For this review, use the dimensioned drawing (mm, ordinates from the lowest corner) and the shaded views. A direction names the side the tool comes from. Give positions to 0.01 mm unless a question says otherwise; leave off trailing zeros. Write each loop counter-clockwise with the first axis right and the second up, starting at its lowest first coordinate (ties: lowest second). Pieces come first, ordered by that corner, then holes.
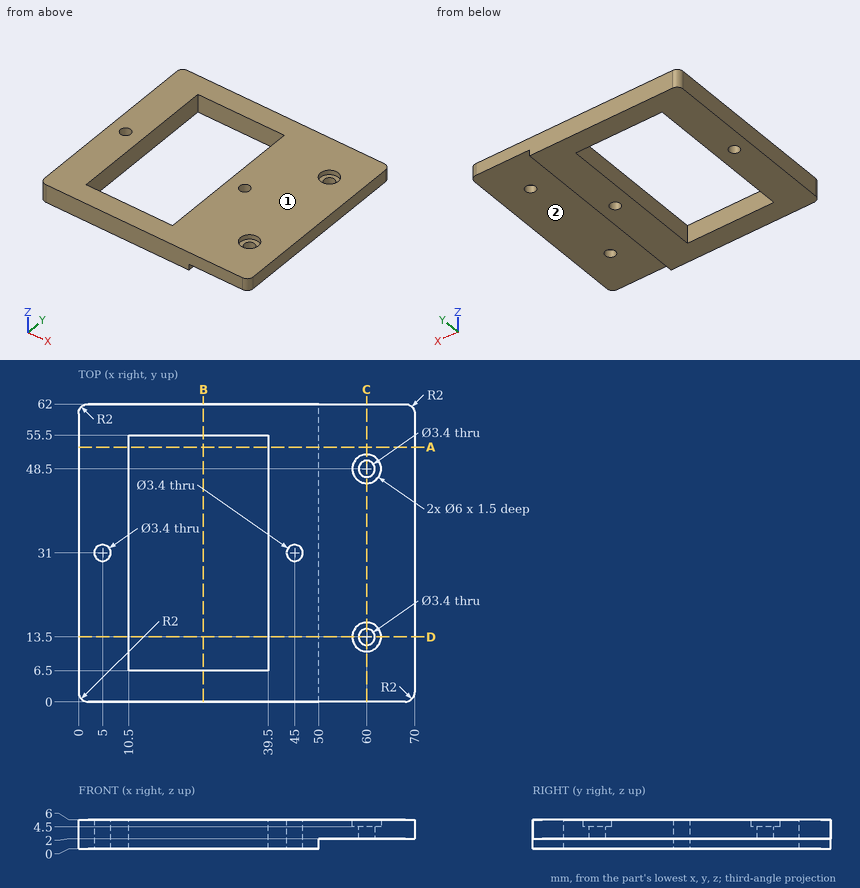
(1) We need section A-A (y = 53). Write out the cut boundary in (x, z), and give its area (3 significant figures).
(2) Tool access review of the marked faces 1 and 2: name each direction out of +Z, -Z, +X, -X, +Y, -Y from which nothing blocks a thin tool from reaching the whole face with its end or side.
(3) Clearance check with flat-ended pins moving along their axes: pin 1 Ø4.5 at (x, y) = (60, 13.5) entering from -Z; pin 2 Ø0.6 at (y, z) = (17.5, 0.5) entering from +X; pin 3 Ø1.8 at (x, y) = (61, 13) entering from +Z; pin 4 Ø3 at (x, y) = (5, 31) entering from -Z. State where each tip first meets the part, or that it passes through.
(4) For L1, parallel to Y at x = 60, z = 2.5; L2, parallel to Y at x = 60, z = 4.95; L3, parallel to Y at x = 27.5, z = 5.35, list the stretches that pass through material, from the lowest coordinate up.
(5) We need section B-B (x = 26). Write out the cut boundary in (y, z), and give its area (3 significant figures).
(6) We need section C-C (x = 60). Write out the cut boundary in (y, z).
(7) We need section D-D (y = 13.5). Write out the cut boundary in (x, z).
The answers:
1. outline: (0, 0) - (10.5, 0) - (10.5, 6) - (0, 6) - close; (39.5, 0) - (50, 0) - (50, 2) - (70, 2) - (70, 6) - (39.5, 6) - close
1. area: 206 mm2
2. face 1: +Z, +X, -X, +Y, -Y
2. face 2: -Z, +X, +Y, -Y
3. pin 1: stops at z = 2
3. pin 2: stops at x = 50
3. pin 3: stops at z = 4.5
3. pin 4: passes through
4. L1: y = 0 to 11.8, 15.2 to 46.8, 50.2 to 62
4. L2: y = 0 to 10.5, 16.5 to 45.5, 51.5 to 62
4. L3: y = 0 to 6.5, 55.5 to 62
5. outline: (0, 0) - (6.5, 0) - (6.5, 6) - (0, 6) - close; (55.5, 0) - (62, 0) - (62, 6) - (55.5, 6) - close
5. area: 78.0 mm2
6. outline: (0, 2) - (11.8, 2) - (11.8, 4.5) - (10.5, 4.5) - (10.5, 6) - (0, 6) - close; (15.2, 2) - (46.8, 2) - (46.8, 4.5) - (45.5, 4.5) - (45.5, 6) - (16.5, 6) - (16.5, 4.5) - (15.2, 4.5) - close; (50.2, 2) - (62, 2) - (62, 6) - (51.5, 6) - (51.5, 4.5) - (50.2, 4.5) - close
7. outline: (0, 0) - (10.5, 0) - (10.5, 6) - (0, 6) - close; (39.5, 0) - (50, 0) - (50, 2) - (58.3, 2) - (58.3, 4.5) - (57, 4.5) - (57, 6) - (39.5, 6) - close; (61.7, 2) - (70, 2) - (70, 6) - (63, 6) - (63, 4.5) - (61.7, 4.5) - close
